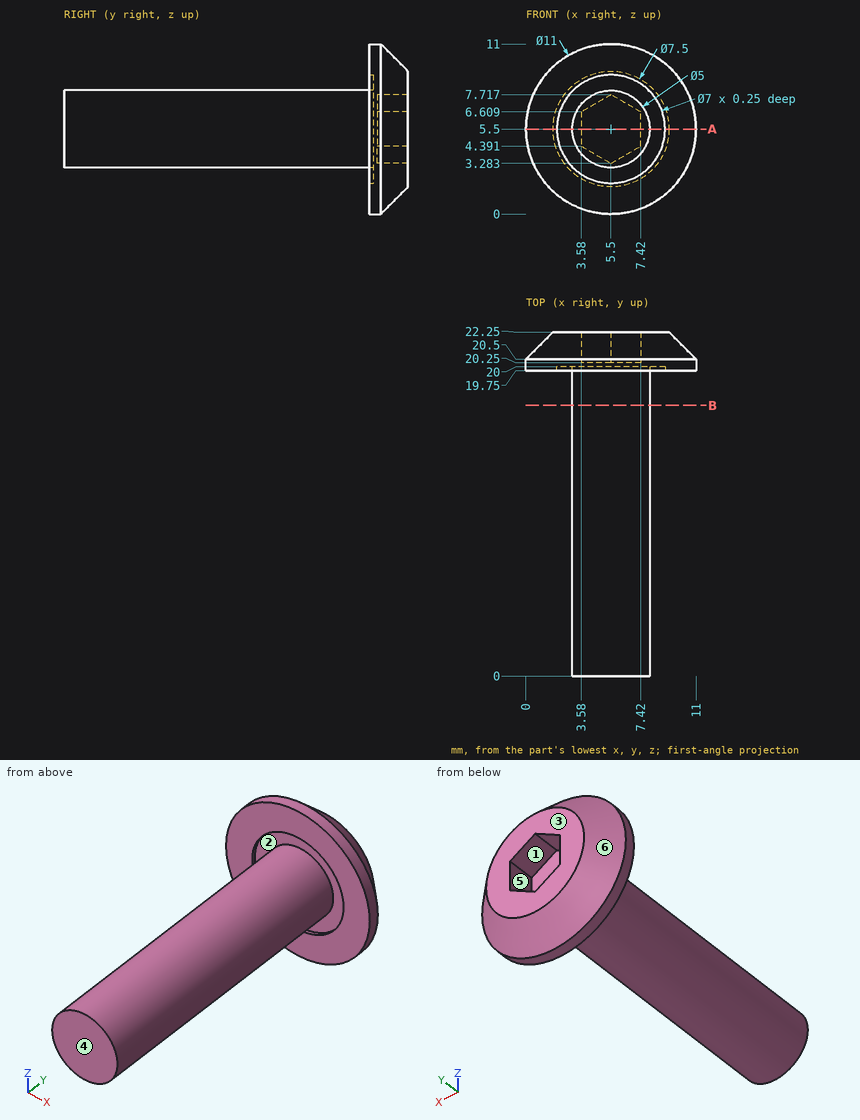
Could you check a few things on this drawing? It's one solid part, dimensions in mm from its lowest x, y, z. A direction names the side the tool comes from. Coordinates: 2 decimals unless noted, no trailing zeros. Write each loop counter-clockwise with the first axis right and the second up, starting at its lowest first coordinate (ties: lowest second). Pieces come first, ordered by that corner, then holes. Notation, with made-up numbers: M 44,77.25 L 74,77.25 A24 ccw 74,108.25 Z; hole C 3,23.5 d11. An arc over 180 degrees is marked long. Answer as CSV lines item,"result". Start each with the question number.
Q1. For the marked faces 1, 2 and 3, which set-ups out of +Z, -Z, +X, -X, +Y, -Y let a thin tool reach every point of the face, with its end or its side?
Q2. Will these pins go through, and if not, where does the flat tip stop? pin 1 Ø1 at (x, y) = (4, 6.5) entering from +Z; pin 2 Ø5 at (x, y) = (2, 19.5) entering from +Z; pin 3 Ø1.6 at (y, z) = (21.5, 5) entering from +X.
Q3. I need wall thicknesses on probe 1 along Z at (x, y) = (5.5, 19.8); probe 2 along Y at (x, z) = (2.25, 6.25); probe 3 along Y at (x, z) = (7, 4.5). Which ranges of each line are inside material? Lowest first, please. Write a range as [from, to].
Q4. Suppose I cut it at A-A, the plane z = 5.5. List the corners of the cut face in (x, y) for me, then the cut area to 3 significant figures.
Q5. Suppose I cut it at B-B, the plane y = 17.5. List the corners of the cut face in (x, z) for me.
Q6. If we mould it in two halves opening along X, with no side actions, what happens to the marked faces 4, 5 and 6? For each: pulls with the +X half, pulls with the -X half, needs draft (parallel to the pull), parting line crosses it, or undercut.
Entries:
1,face 1,"+Y"
1,face 2,"-Y"
1,face 3,"+Z, -Z, +X, -X, +Y"
2,pin 1,"stops at z = 7.79"
2,pin 2,"stops at z = 10.91"
2,pin 3,"stops at x = 10.78"
3,probe 1,"z = [0, 2], [3, 8], [9, 11]"
3,probe 2,"y = [20, 22.25]"
3,probe 3,"y = [0, 20.25]"
4,outline,"M 0,19.75 L 2,19.75 L 2,20 L 3,20 L 3,0 L 8,0 L 8,20 L 9,20 L 9,19.75 L 11,19.75 L 11,20.5 L 9.25,22.25 L 7.42,22.25 L 7.42,20.25 L 3.58,20.25 L 3.58,22.25 L 1.75,22.25 L 0,20.5 Z"
4,area,"115 mm²"
5,outline,"C 5.5,5.5 d5"
6,face 4,"needs draft"
6,face 5,"undercut"
6,face 6,"parting line crosses it"
